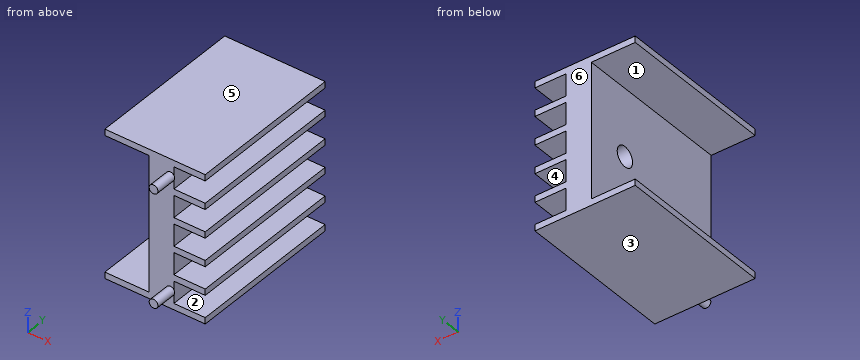
from build123d import *

# Parameters (mm, degrees)
SKETCH1_W           = 4
SKETCH1_H           = 23.5
BOSS_EXTRUDE1_DEPTH = 25
SKETCH2_W           = 5
SKETCH2_H           = 1
SKETCH2_W_2         = 7
BOSS_EXTRUDE2_DEPTH = 25
SKETCH3_R           = 1.6
CUT_EXTRUDE1_DEPTH  = 25
SKETCH4_R           = 0.7
BOSS_EXTRUDE3_DEPTH = 3.5


with BuildPart() as part:
    # Sketch1 → Boss-Extrude1 (new body)
    with BuildSketch(Plane(origin=(0, 0, 0), x_dir=(1, 0, 0), z_dir=(0, 1, 0))):
        Rectangle(SKETCH1_W, SKETCH1_H)
    extrude(amount=BOSS_EXTRUDE1_DEPTH)

    # Sketch2 → Boss-Extrude2 (add)
    with BuildSketch(Plane(origin=(0, 25, 0), x_dir=(1, 0, 0), z_dir=(0, 1, 0))):
        with Locations((4.5, -11.25)):
            Rectangle(SKETCH2_W, SKETCH2_H)
        with Locations((-5.5, -11.25)):
            Rectangle(SKETCH2_W_2, SKETCH2_H)
        with Locations((-5.5, 11.25)):
            Rectangle(SKETCH2_W_2, SKETCH2_H)
        with Locations((4.5, 11.25)):
            Rectangle(SKETCH2_W, SKETCH2_H)
        with Locations((4.5, 6.75)):
            Rectangle(SKETCH2_W, SKETCH2_H)
        with Locations((4.5, 2.25)):
            Rectangle(SKETCH2_W, SKETCH2_H)
        with Locations((4.5, -2.25)):
            Rectangle(SKETCH2_W, SKETCH2_H)
        with Locations((4.5, -6.75)):
            Rectangle(SKETCH2_W, SKETCH2_H)
    extrude(amount=-BOSS_EXTRUDE2_DEPTH)

    # Sketch3 → Cut-Extrude1 (cut)
    with BuildSketch(Plane.ZY.offset(2)):
        with Locations((0, 18)):
            Circle(SKETCH3_R)
    extrude(amount=-CUT_EXTRUDE1_DEPTH, mode=Mode.SUBTRACT)

    # Sketch4 → Boss-Extrude3 (add)
    with BuildSketch(Plane.XZ):
        with Locations(Location((1.43876577, 9, 0), (0, 0, 36.701194363))):
            Circle(SKETCH4_R)
        with Locations(Location((1.43876577, -9, 0), (0, 0, 36.701194363))):
            Circle(SKETCH4_R)
    extrude(amount=BOSS_EXTRUDE3_DEPTH)


solid = part.part
Input: part model. Units: mm. Frame: model coordinates. Face numbers are marked on the shaded views. A direction names the side the tool comes from. Round coordinates to 2 decimals unless told otherwise and drop trailing zeros. Write each loop counter-clockwise with the first axis right and the second up, starting at its lowest first coordinate (ties: lowest second). Pieces come first, ordered by that corner, then holes.
1) Cut plane A-A (z = 0). Return the cut outline in (x, y).
2) Cut plane D-D (x = 4). Return the cut outline in (y, z), then the cut area to 3 significant figures.
3) Ray query, L1, parallel to Z at x = 4, y = 15; L2, parallel to Z at x = -3, y = 8; L3, parallel to Y at x = -0.95, z = 0. Return the intervals inside material, ascending.
4) Draft query along Z for the marked faces 4, 5 and 6. Return one class per face: pulls with the +Z half, pulls with the -Z half, needs draft (parallel to the pull), parting line crosses it, or undercut.
5) Contact query for flat-ended pins moving along their axis: P1, Ø1.5, axis at x = -5.5, z = 9, coming from the +Y side; P2, Ø1.8, axis at y = 11, z = 9.5, coming from the +X side; P3, Ø6.5, axis at y = 13, z = -4, coming from the -X side. Output: stop coordinate, or through.
6) Reachability of the marked faces 1, 2 and 3 from +Z, -Z, +X, -X, +Y, -Y: full face, straight path, thin tool, end or side. Return the list, or none.
7) Cut plane B-B (x = -7). Return the cut outline in (y, z), then the cut area to 3 significant figures.
Geometry says:
1. outline: (-2, 0) - (2, 0) - (2, 16.4) - (-2, 16.4) - close; (-2, 19.6) - (2, 19.6) - (2, 25) - (-2, 25) - close
2. outline: (0, -11.75) - (25, -11.75) - (25, -10.75) - (0, -10.75) - close; (0, -7.25) - (25, -7.25) - (25, -6.25) - (0, -6.25) - close; (0, -2.75) - (25, -2.75) - (25, -1.75) - (0, -1.75) - close; (0, 1.75) - (25, 1.75) - (25, 2.75) - (0, 2.75) - close; (0, 6.25) - (25, 6.25) - (25, 7.25) - (0, 7.25) - close; (0, 10.75) - (25, 10.75) - (25, 11.75) - (0, 11.75) - close
2. area: 150 mm2
3. L1: z = -11.75 to -10.75, -7.25 to -6.25, -2.75 to -1.75, 1.75 to 2.75, 6.25 to 7.25, 10.75 to 11.75
3. L2: z = -11.75 to -10.75, 10.75 to 11.75
3. L3: y = 0 to 16.4, 19.6 to 25
4. face 4: undercut
4. face 5: pulls with the +Z half
4. face 6: needs draft
5. P1: passes through
5. P2: stops at x = 2
5. P3: stops at x = -2
6. face 1: -X, +Y, -Y
6. face 2: +X, +Y, -Y
6. face 3: -Z, +X, -X, +Y, -Y
7. outline: (0, -11.75) - (25, -11.75) - (25, -10.75) - (0, -10.75) - close; (0, 10.75) - (25, 10.75) - (25, 11.75) - (0, 11.75) - close
7. area: 50.0 mm2
